```python
from build123d import *

# Parameters (mm, degrees)
SKETCH7_R           = 6.5
BOSS_EXTRUDE2_DEPTH = 0.396875
FILLET1_R           = 0.79375
SKETCH6_R           = 6
BOSS_EXTRUDE1_DEPTH = 5
SKETCH5_R           = 1.651
CUT_EXTRUDE3_DEPTH  = 8.89


with BuildPart() as part:
    # Sketch2 → Revolve1 (revolve)
    with BuildSketch(Plane.XY):
        with BuildLine():
            Line((0, 0), (0, -2.38125))
            Line((0, -2.38125), (12.7, -2.38125))
            Line((12.7, -2.38125), (12.7, -1.374815329))
            ThreePointArc((12.7, -1.374815329), (11.90625, 0), (12.7, 1.374815329))
            Line((12.7, 1.374815329), (12.7, 2.38125))
            Line((12.7, 2.38125), (0, 2.38125))
            Line((0, 2.38125), (0, 0))
        make_face()
    revolve(axis=Axis((0, 0, 0), (0, 1, 0)))

    # Sketch7 → Boss-Extrude2 (add)
    with BuildSketch(Plane(origin=(0, -2.38125, 0), x_dir=(-1, 0, 0), z_dir=(0, -1, 0))):
        with Locations(Location((0, 0, 0), (0, 0, 180))):
            Circle(SKETCH7_R)
    extrude(amount=BOSS_EXTRUDE2_DEPTH)

    # Fillet1
    # the kernel refuses this fillet: 0.79375 mm, written as the material it adds along each edge
    with BuildSketch(Plane(origin=(0, -2.38125, 0), x_dir=(1, 0, 0), z_dir=(0, 0, -1))) as fillet1_piece_1:
        with BuildLine():
            CenterArc((7.187407664, 0.79375), FILLET1_R, 210, 60)
            Line((6.5, 0.396875), (6.486251847, 0.3889375))
            ThreePointArc((6.486251847, 0.3889375), (6.484125, 0.1984375), (6.484125, 0))
            Line((6.484125, 0), (6.5, -0.015875))
            Line((6.5, -0.015875), (7.187407664, -0.015875))
            Line((7.187407664, -0.015875), (7.187407664, 0))
        make_face()
    revolve(axis=Axis((0, -2.38125, 0), (0, -1, 0)))

    # Sketch6 → Boss-Extrude1 (add)
    with BuildSketch(Plane.XZ.offset(2.778125)):
        Circle(SKETCH6_R)
    extrude(amount=BOSS_EXTRUDE1_DEPTH)

    # Sketch5 → Cut-Extrude3 (cut)
    with BuildSketch(Plane.XZ.offset(7.778125)):
        with Locations((-1.7145, 0)):
            Circle(SKETCH5_R)
        with Locations((1.7145, 0)):
            Circle(SKETCH5_R)
    extrude(amount=-CUT_EXTRUDE3_DEPTH, mode=Mode.SUBTRACT)


solid = part.part
```
Input: part model. Units: mm. Frame: model coordinates. A direction names the side the tool comes from. Give positions to 0.01 mm unless a question says otherwise; leave off trailing zeros. Order: outer loops, then holes, each group sorted by start corner. A loop starts at its lowest first (then second) coordinate and runs counter-clockwise, first axis right, second up. Notation, with made-up numbers: (-7.75, -26) - (22.25, -26) arc R16 ccw to (22.25, 3) - close; hole circle Ø3 at (-33.5, -8). An arc over 180 degrees is marked (long way). Put each result on its own line as item: value.
Item 1: Contact query for flat-ended pins moving along their axis: pin 1 (2 mm diameter, centred on y = -3.5, z = -8, fed in from -X); pin 2 (2.5 mm diameter, centred on x = -1.5, z = 0, fed in from -Y); pin 3 (4 mm diameter, centred on y = -2.5, z = 7, fed in from +X); pin 4 (1 mm diameter, centred on x = -2.5, y = -1, fed in from -Z). Output: stop coordinate, or through.
Found:
pin 1: passes through
pin 2: stops at y = 1.11
pin 3: stops at x = 11.67
pin 4: stops at z = -12.51
Item 2: Section query C-C, the plane y = -4.25. Return loops of the section in (x, z), then the cut area to 3 significant figures.
Found:
outline: circle Ø12 at (0, 0); hole circle Ø3.3 at (-1.71, 0); hole circle Ø3.3 at (1.71, 0)
area: 96.0 mm^2
Item 3: Ray query, L1, parallel to Y at x = 0.75, z = -6; L2, parallel to Y at x = 8.25, z = 1.5; L3, parallel to Y at x = -6.5, z = 10.25. Return the intervals inside material, ascending. Write a range as from..to.
Found:
L1: y = -2.78..2.38
L2: y = -2.38..2.38
L3: y = -2.38..-0.82, 0.82..2.38
Item 4: Section query B-B, the plane y = 1.75. Return loops of the section in (x, z), then the cut area to 3 significant figures.
Found:
outline: circle Ø25.4 at (0, 0)
area: 507 mm^2
Item 5: Access query for faces 1 (the cylindrical face through (-6, -5, 0)), 2 (the flat face through (0, 2.381, 0)). Directions: +Z, -Z, +X, -X, +Y, -Y. A direction counts if a zero-diameter tool reaches every point of the face in a straight line with its end or side. Return the directions, or none.
Found:
face 1: -Y
face 2: +Z, -Z, +X, -X, +Y
Item 6: Draft query along X for faces 3 (the flat face through (-2, 1.112, 0)), 4 (the cylindrical face through (-2.75, -1.87, 12.4)), 5 (the cylindrical face through (-3.364, -3.395, 0.073)), 6 (the flat face through (0, -7.778, -1)). Return one class per face: +X half, -X half, draft (parallel to the pull), parting line (faces both ways), or undercut.
Found:
face 3: undercut
face 4: parting line
face 5: undercut
face 6: draft
